Solid Edge part; units mm, degrees
sketch "Sketch1" plane through (0, 0, 0) normal (0, -1, 0) x (1, 0, 0)
  line L0 (17, 21) -> (-17, 21)
  arc A0 (-17, 21) -> (-21, 17) centre (-17, 17) ccw
  line L1 (-21, 17) -> (-21, -17)
  arc A1 (-21, -17) -> (-17, -21) centre (-17, -17) ccw
  line L2 (-17, -21) -> (17, -21)
  arc A2 (17, -21) -> (21, -17) centre (17, -17) ccw
  line L3 (21, -17) -> (21, 17)
  arc A3 (21, 17) -> (17, 21) centre (17, 17) ccw
  arc A4 (-17, 25) -> (-25, 17) centre (-17, 17) ccw
  line L4 (-25, 17) -> (-25, -17)
  arc A5 (-25, -17) -> (-17, -25) centre (-17, -17) ccw
  line L5 (-17, -25) -> (17, -25)
  arc A6 (17, -25) -> (25, -17) centre (17, -17) ccw
  line L6 (25, -17) -> (25, 17)
  arc A7 (25, 17) -> (17, 25) centre (17, 17) ccw
  line L7 (17, 25) -> (-17, 25)
extrude "Protrusion1" add sketch "Sketch1" against normal blind 38.1
CAD build for the part. Positions are in the model's coordinates, mm. A direction names the side the tool comes from. Coordinates: 2 decimals unless noted, no trailing zeros. Loops run counter-clockwise (first coordinate to the right, second up) from the corner with the lowest first, then second, coordinate; pieces in that order, holes last. Notation, with made-up numbers: (-9, 78.25) - (1, 78.25) arc R13 cw to (1, 87.25) - close; hole circle Ø11 at (26.5, 68). An arc over 180 degrees is marked (long way). Use one line per item in the form item = value. Start each with the question number.
1) Flat gauge pin, fed straight in: pin 1 (8 mm diameter, centred on x = 19, z = -4.5, fed in from +Y). Where does the tip first touch, or does it go through?
2) Band-saw the part on C-C (y = 5). Give the cut face in (x, z), and give its area (3 significant figures).
3) Two-plate mould, pull along X, no slides. Class faces 1 (the face through (0, 38.1, 23)), 2 (the face through (22.719, 18.783, 22.594)), 3 (the face through (0, 19, 21)): +X half, -X half, draft (parallel to the pull), parting line (faces both ways), or undercut.
4) Band-saw the part on B-B (z = 12.5). Give the cut face in (x, y), and give its area (3 significant figures).
5) Band-saw the part on A-A (x = 1). Give the cut face in (y, z).
6) Band-saw the part on D-D (x = -22). Give the cut face in (y, z) (3 decimals), and give its area (3 significant figures).
7) Tool access for faces 4 (the face through (25, 19, 0)), 5 (the face through (21, 19, 0)): list every direction of +Z, -Z, +X, -X, +Y, -Y with a clear straight run to the whole face (end or side of a thin tool).
8) Drill centre lines: L1, parallel to Z at x = -13, y = 7; L2, parallel to X at y = 16, z = -18. Where is each one in solid material? Low to high. Write a range as from..to.
Check values:
q1.pin_1 = 38.1
q2.outline = (-25, -17) arc R8 ccw to (-17, -25) - (17, -25) arc R8 ccw to (25, -17) - (25, 17) arc R8 ccw to (17, 25) - (-17, 25) arc R8 ccw to (-25, 17) - close; hole (-21, -17) arc R4 ccw to (-17, -21) - (17, -21) arc R4 ccw to (21, -17) - (21, 17) arc R4 ccw to (17, 21) - (-17, 21) arc R4 ccw to (-21, 17) - close
q2.area = 695 mm2
q3.face_1 = draft
q3.face_2 = +X half
q3.face_3 = undercut
q4.outline = (-25, 0) - (-21, 0) - (-21, 38.1) - (-25, 38.1) - close; (21, 0) - (25, 0) - (25, 38.1) - (21, 38.1) - close
q4.area = 305 mm2
q5.outline = (0, -25) - (38.1, -25) - (38.1, -21) - (0, -21) - close; (0, 21) - (38.1, 21) - (38.1, 25) - (0, 25) - close
q6.outline = (0, -23.245) - (38.1, -23.245) - (38.1, 23.245) - (0, 23.245) - close
q6.area = 1,770 mm2
q7.face_4 = +Z, -Z, +X, +Y, -Y
q7.face_5 = +Y, -Y
q8.L1 = -25..-21, 21..25
q8.L2 = -24.94..-20.87, 20.87..24.94
